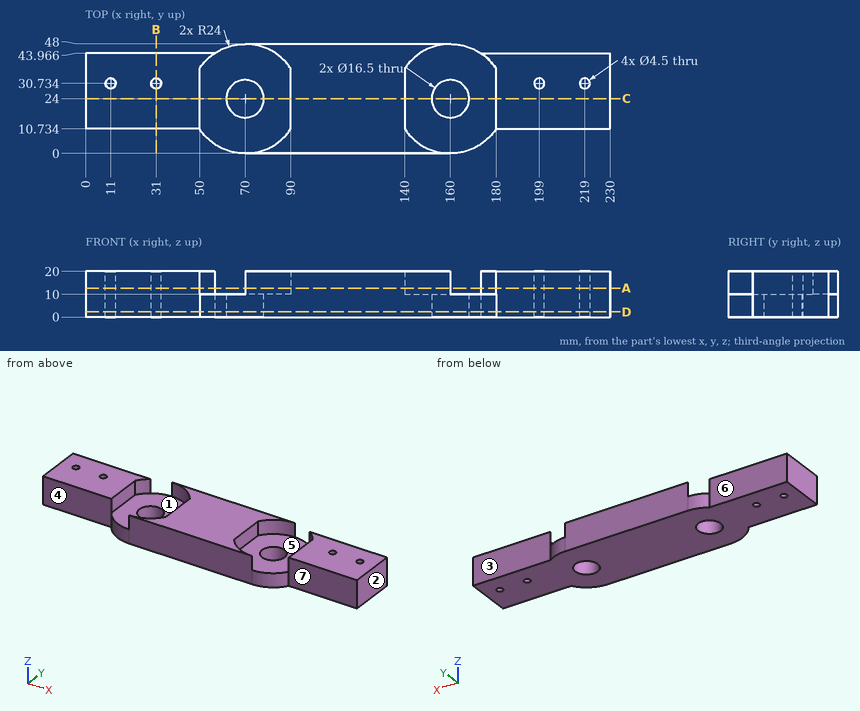
Design review of the part shown in the three views and the two pictorial views. Dimensions are in mm from the part's minimum x, y and z. A direction names the side the tool comes from. Round coordinates to 2 decimals unless told otherwise and drop trailing zeros. Write each loop counter-clockwise with the first axis right and the second up, starting at its lowest first coordinate (ties: lowest second). Pieces come first, ordered by that corner, then holes. Notation, with made-up numbers: M 68,38.5 L 94,38.5 A16 ccw 94,42.5 Z; hole C -1,-21 d8. An arc over 180 degrees is marked long. Use a Markdown table: item, result. Add a question column.
Q1. Machinability: for the marked faces 4, 5, 6 and 7, which of the approach directions +Z, -Z, +X, -X, +Y, -Y give a long, thin tool a straight path to every point of the face, cutting with its end or side? Answer none if there is none.
Q2. We need section C-C, the plane y = 24. State the section outline as (x, z) points.
Q3. We need section A-A, the plane z = 12.75. State the section outline as (x, y) points.
Q4. The part is to be moulded in two halves that separate along Y. For the marked faces 1, 2 and 3, say which applies: pulls with the +Y half, pulls with the -Y half, needs draft (parallel to the pull), parting line crosses it, or undercut.
Q5. We need section B-B, the plane x = 31. State the section outline as (y, z) points, plus the area to 3 significant figures.
Q6. Insertion check: pin 1 (10 mm diameter, centred on x = 201.5, z = 14, fed in from +Y); pin 2 (12 mm diameter, centred on x = 169.5, z = 2, fed in from +Y); pin 3 (6 mm diameter, centred on x = 194, z = 10.5, fed in from -Y). Each pin has a flat end and moves straight along its axis. Give the tip position at first contact, or say it passes through.
Q7. To check wall thickness, follow line 1 (X direction, y = 13, z = 16); line 2 (Y direction, x = 11, z = 9.5); line 3 (Y direction, x = 70, z = 6.25). State the ranges of each line that lie inside material, in increasing order.
Q8. We need section D-D, the plane z = 2.25. State the section outline as (x, y) points, plus the area to 3 significant figures.
Findings below:
| question | item | result |
|---|---|---|
| 1 | face 4 | +Z, -Z, -X, -Y |
| 1 | face 5 | +Z |
| 1 | face 6 | +Z, -Z, -X, +Y |
| 1 | face 7 | +Z, -Z, +X, -Y |
| 2 | outline | M 0,0 L 61.75,0 L 61.75,10 L 50,10 L 50,20 L 0,20 Z; M 78.25,0 L 151.75,0 L 151.75,10 L 140,10 L 140,20 L 90,20 L 90,10 L 78.25,10 Z; M 168.25,0 L 230,0 L 230,20 L 180,20 L 180,10 L 168.25,10 Z |
| 3 | outline | M 0,10.73 L 50,10.73 L 50,37.27 A24 cw 56.68,43.97 L 0,43.97 Z; M 70,0 L 160,0 A24 cw 140,10.73 L 140,37.27 A24 cw 160,48 L 70,48 A24 cw 90,37.27 L 90,10.73 A24 cw Z; M 173.32,43.97 A24 cw 180,37.27 L 180,10.73 L 230,10.73 L 230,43.97 Z; hole C 11,30.73 d4.5; hole C 31,30.73 d4.5; hole C 199,30.73 d4.5; hole C 219,30.73 d4.5 |
| 4 | face 1 | undercut |
| 4 | face 2 | needs draft |
| 4 | face 3 | pulls with the +Y half |
| 5 | outline | M 10.73,0 L 28.48,0 L 28.48,20 L 10.73,20 Z; M 32.98,0 L 43.97,0 L 43.97,20 L 32.98,20 Z |
| 5 | area | 575 mm² |
| 6 | pin 1 | stops at y = 43.97 |
| 6 | pin 2 | stops at y = 47.74 |
| 6 | pin 3 | stops at y = 10.73 |
| 7 | line 1 | x = 0 to 50, 90 to 140, 180 to 230 |
| 7 | line 2 | y = 10.73 to 28.48, 32.98 to 43.97 |
| 7 | line 3 | y = 0 to 15.75, 32.25 to 48 |
| 8 | outline | M 0,10.73 L 50,10.73 A24 ccw 70,0 L 160,0 A24 ccw 180,10.73 L 230,10.73 L 230,43.97 L 173.32,43.97 A24 ccw 160,48 L 70,48 A24 ccw 56.68,43.97 L 0,43.97 Z; hole C 11,30.73 d4.5; hole C 31,30.73 d4.5; hole C 70,24 d16.5; hole C 160,24 d16.5; hole C 199,30.73 d4.5; hole C 219,30.73 d4.5 |
| 8 | area | 8,860 mm² |
